Can you work these out from the model? Positions are in its coordinate system, mm. Coordinates: 2 decimals unless noted, no trailing zeros. Loops run counter-clockwise (first coordinate to the right, second up) from the corner with the lowest first, then second, coordinate; pieces in that order, holes last.
```python
from build123d import *

# Parameters (mm, degrees)
SKETCH_1_W          = 90
SKETCH_1_H          = 63
EXTRUDE_1_DEPTH     = 2
SKETCH_2_W          = 79
SKETCH_2_H          = 51
EXTRUDE_2_DEPTH     = 5
SKETCH_3_R          = 1
CUT_EXTRUDE_1_DEPTH = 75.760510392


with BuildPart() as part:
    # 草图1 → 凸台-拉伸1 (new body)
    with BuildSketch(Plane(origin=(0, 0, 0), x_dir=(1, 0, 0), z_dir=(0, 1, 0))):
        with Locations((14.879032258, -12.981854839)):
            Rectangle(SKETCH_1_W, SKETCH_1_H)
    extrude(amount=EXTRUDE_1_DEPTH)

    # 草图2 → 凸台-拉伸2 (add)
    with BuildSketch(Plane(origin=(0, 2, 0), x_dir=(1, 0, 0), z_dir=(0, 1, 0))):
        with Locations((14.879032258, -12.981854839)):
            Rectangle(SKETCH_2_W, SKETCH_2_H)
    extrude(amount=EXTRUDE_2_DEPTH)

    # 草图3 → 切除-拉伸1 (cut, through all)
    with BuildSketch(Plane(origin=(0, 2, 0), x_dir=(1, 0, 0), z_dir=(0, 1, 0))):
        with Locations(Location((-28.120967742, 16.518145161, 0), (0, 0, 270))):
            Circle(SKETCH_3_R)
        with Locations(Location((-28.120967742, -42.481854839, 0), (0, 0, 270))):
            Circle(SKETCH_3_R)
        with Locations(Location((57.879032258, -42.481854839, 0), (0, 0, 270))):
            Circle(SKETCH_3_R)
        with Locations(Location((57.879032258, 16.518145161, 0), (0, 0, 270))):
            Circle(SKETCH_3_R)
    extrude(amount=-CUT_EXTRUDE_1_DEPTH, mode=Mode.SUBTRACT)


solid = part.part
```
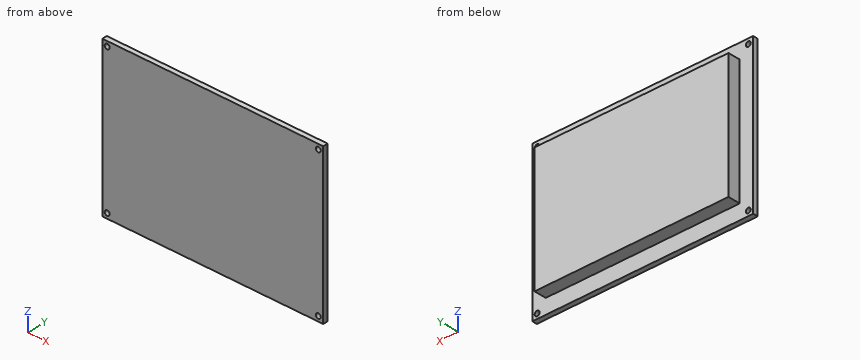
(1) I want a section at D-D on z = 40.5. Write out the boundary of the cut face in (x, y).
Check values:
outline: (-30.12, 0) - (59.88, 0) - (59.88, 2) - (-30.12, 2) - close
(2) I want a section at B-B on z = 7.5. Write out the boundary of the cut face in (x, y), then the cut area to 3 significant figures.
Check values:
outline: (-30.12, 0) - (59.88, 0) - (59.88, 2) - (54.38, 2) - (54.38, 7) - (-24.62, 7) - (-24.62, 2) - (-30.12, 2) - close
area: 575 mm2
(3) I want a section at C-C on y = 5.25. Write out the boundary of the cut face in (x, z), then the cut area to 3 significant figures.
Check values:
outline: (-24.62, -12.52) - (54.38, -12.52) - (54.38, 38.48) - (-24.62, 38.48) - close
area: 4,030 mm2
(4) If I drill on probe 1 along Z at (x, y) = (8.5, 3.75); probe 2 along Y at (x, z) = (16.5, 40); probe 3 along X at (y, z) = (6.5, -5), over which ranges is the centre line in solid material (lowest first)?
Check values:
probe 1: z = -12.52 to 38.48
probe 2: y = 0 to 2
probe 3: x = -24.62 to 54.38
(5) I'm going to push flat-ended pins straight in: pin 1 (3 mm diameter, centred on x = 57.88, z = -16.52, fed in from +Y); pin 2 (1 mm diameter, centred on x = -17, y = 3, fed in from -Z); pin 3 (2.5 mm diameter, centred on y = 4, z = 22, fed in from +X). Where does each tip first touch, or does it pass through?
Check values:
pin 1: stops at y = 2
pin 2: stops at z = -12.52
pin 3: stops at x = 54.38
(6) I want a section at A-A on x = 7. Write out the boundary of the cut face in (y, z).
Check values:
outline: (0, -18.52) - (2, -18.52) - (2, -12.52) - (7, -12.52) - (7, 38.48) - (2, 38.48) - (2, 44.48) - (0, 44.48) - close
